Work out the finished part from the listing and answer in its coordinate system (mm). A direction names the side the tool comes from. Coordinates: 2 decimals unless noted, no trailing zeros. Order: outer loops, then holes, each group sorted by start corner. A loop starts at its lowest first (then second) coordinate and runs counter-clockwise, first axis right, second up. Notation, with made-up numbers: M 78,78 L 131,78 A36 ccw 131,112 Z; hole C 24.5,-8.5 d9. An arc over 180 degrees is marked long. Use a Markdown table: item, result.
from build123d import *

# Parameters (mm, degrees)
SKETCH1_R           = 31.35
SKETCH1_R_2         = 16.65
BOSS_EXTRUDE1_DEPTH = 3
SKETCH2_R           = 4.85
BOSS_EXTRUDE2_DEPTH = 18
CIRPATTERN1_COUNT   = 6
CHAMFER1_SIZE       = 0.6
SCALE1_SCALE        = 0.4


with BuildPart() as part:
    # Sketch1 → Boss-Extrude1 (new body)
    with BuildSketch(Plane.XY):
        Circle(SKETCH1_R)
        Circle(SKETCH1_R_2, mode=Mode.SUBTRACT)
    extrude(amount=-BOSS_EXTRUDE1_DEPTH)

    # Sketch2 → Boss-Extrude2 (add)
    with BuildSketch(Plane.XY):
        with Locations((24, 0)):
            Circle(SKETCH2_R)
    boss_extrude2 = extrude(amount=BOSS_EXTRUDE2_DEPTH)

    # CirPattern1: Boss-Extrude2 ×6 about axis
    cirpattern1_axis = Axis((0, 0, 0), (0, 0, 1))
    for i in range(1, CIRPATTERN1_COUNT):
        add(boss_extrude2.rotate(cirpattern1_axis, i * 360 / CIRPATTERN1_COUNT))

    # Chamfer1
    chamfer1_edges = [part.edges().sort_by_distance(p)[0] for p in [
        (19.15, 0, 18),
        (9.575, -16.584386482, 18),
        (-9.575, -16.584386482, 18),
        (-31.35, 0, 0),
        (-19.15, 0, 18),
        (-9.575, 16.584386482, 18),
        (9.575, 16.584386482, 18),
        (-31.35, 0, -3),
        (-16.65, 0, -3),
        (-16.65, 0, 0),
    ]]
    chamfer(chamfer1_edges, length=CHAMFER1_SIZE)


with BuildPart() as part_1:
    # Scale1: scaled about (0, 0, 4.240913614)
    add(part.part.scale(SCALE1_SCALE).moved(Location((0, 0, 2.544548168))))


solid = part_1.part
(1) Which of the six approach directions +Z, -Z, +X, -X, +Y, -Y give full straight-line access (tool end or side, diameter ignored) to faces 4 (the flat face through (-10, 0, 9.745)), 5 (the cylindrical face through (11.392, -0.743, 5.976))?
Conclusion:
| item | result |
|---|---|
| face 4 | +Z, +X, -X, +Y, -Y |
| face 5 | +Z |
(2) A cutting plane is placed at B-B (z = 2). Determine the outline of the cut face in (x, y).
Conclusion:
| item | result |
|---|---|
| outline | C 0,0 d25.08; hole C 0,0 d13.32 |
(3) Given P1, Ø3, axis at x = 6, y = 0.5, coming from the +Z side; P2, Ø5, axis at y = 1.5, z = 6.5, coming from the -X side; P3, Ø2, axis at x = -6.5, z = 6, coming from the +Y side, each flat-ended and moving along its own axis, determine where each tip first touches the part or whether it passes through.
Conclusion:
| item | result |
|---|---|
| P1 | z = 2.54 |
| P2 | x = -11.54 |
| P3 | y = 10.12 |
(4) Determine the mould class of faces 1 (the flat face through (5, 8, 9.745)), 2 (the cylindrical face through (-9.24, 8.48, 1.95)), 3 (the cylindrical face through (-2.95, -7.73, 5.98)) for opening direction Y: pulls with the +Y half, pulls with the -Y half, needs draft (parallel to the pull), parting line crosses it, or undercut.
Conclusion:
| item | result |
|---|---|
| face 1 | needs draft |
| face 2 | parting line crosses it |
| face 3 | undercut |
(5) Straight lines are drawn through the part: L1, parallel to Y at x = 0, z = 2.1; L2, parallel to Z at x = -1, y = -8.5; L3, parallel to Y at x = -2.75, z = 2. For each, find the intervals that lie inside material, in ascending order.
Conclusion:
| item | result |
|---|---|
| L1 | -12.54 to -6.66, 6.66 to 12.54 |
| L2 | 1.34 to 2.54 |
| L3 | -12.23 to -6.07, 6.07 to 12.23 |
(6) A cutting plane is placed at A-A (y = 0). Determine the outline of the cut face in (x, z), then the cut area to 3 significant figures.
Conclusion:
| item | result |
|---|---|
| outline | M -12.54,1.58 L -12.3,1.34 L -6.9,1.34 L -6.66,1.58 L -6.66,2.3 L -6.9,2.54 L -7.66,2.54 L -7.66,9.5 L -7.9,9.74 L -11.3,9.74 L -11.54,9.5 L -11.54,2.54 L -12.3,2.54 L -12.54,2.3 Z; M 6.66,1.58 L 6.9,1.34 L 12.3,1.34 L 12.54,1.58 L 12.54,2.3 L 12.3,2.54 L 11.54,2.54 L 11.54,9.5 L 11.3,9.74 L 7.9,9.74 L 7.66,9.5 L 7.66,2.54 L 6.9,2.54 L 6.66,2.3 Z |
| area | 69.6 mm2 |
